The model under review builds one solid part; all positions refer to its coordinate system, in mm. A direction names the side the tool comes from. Give positions to 0.01 mm unless a question says otherwise; leave off trailing zeros. Loops run counter-clockwise (first coordinate to the right, second up) from the corner with the lowest first, then second, coordinate; pieces in that order, holes last. Notation, with made-up numbers: M 82.5,-11.5 L 114.5,-11.5 A15 cw 114.5,12.5 Z; hole C 15.5,62.25 d1. An arc over 180 degrees is marked long. Put each result on its own line as item: value. Start each with the question number.
```python
from build123d import *

# Parameters (mm, degrees)
BOSS_EXTRUDE1_DEPTH = 5


with BuildPart() as part:
    # Sketch2 → Boss-Extrude1 (new body)
    with BuildSketch(Plane(origin=(0, 0, 0), x_dir=(1, 0, 0), z_dir=(0, 1, 0))):
        with BuildLine():
            Line((-46.361864593, 80.672065662), (46.361864593, 80.672065662))
            Line((46.361864593, 80.672065662), (66.733304285, 94.936301299))
            ThreePointArc((66.733304285, 94.936301299), (74.205550425, 96.592858386), (80.660589091, 92.480545219))
            Line((80.660589091, 92.480545219), (89.264235636, 80.193264555))
            ThreePointArc((89.264235636, 80.193264555), (90.920792724, 72.721018415), (86.808479557, 66.265979749))
            Line((86.808479557, 66.265979749), (62.402393643, 49.176654414))
            ThreePointArc((62.402393643, 49.176654414), (59.268049675, 45.602620103), (58.138158007, 40.985133971))
            Line((58.138158007, 40.985133971), (58.138158007, 16.396474982))
            ThreePointArc((58.138158007, 16.396474982), (57.008266339, 11.77898885), (53.873922371, 8.204954539))
            Line((53.873922371, 8.204954539), (41.764235636, -0.274339397))
            ThreePointArc((41.764235636, -0.274339397), (38.629891668, -3.848373708), (37.5, -8.46585984))
            Line((37.5, -8.46585984), (37.5, -283.0815533))
            ThreePointArc((37.5, -283.0815533), (38.82037806, -288.047856048), (42.432832597, -291.702679358))
            Line((42.432832597, -291.702679358), (110.719624802, -331.839038015))
            ThreePointArc((110.719624802, -331.839038015), (114.964915466, -336.816247945), (115.224929316, -343.352875846))
            Line((115.224929316, -343.352875846), (110.804845639, -357.979679412))
            ThreePointArc((110.804845639, -357.979679412), (105.193270142, -364.269086107), (96.767619692, -364.034926706))
            Line((96.767619692, -364.034926706), (4.46475403, -317.978659754))
            ThreePointArc((4.46475403, -317.978659754), (0, -316.92661882), (-4.46475403, -317.978659754))
            Line((-4.46475403, -317.978659754), (-96.767619692, -364.034926706))
            ThreePointArc((-96.767619692, -364.034926706), (-105.193270142, -364.269086107), (-110.804845639, -357.979679412))
            Line((-110.804845639, -357.979679412), (-115.224929316, -343.352875846))
            ThreePointArc((-115.224929316, -343.352875846), (-114.964915466, -336.816247945), (-110.719624802, -331.839038015))
            Line((-110.719624802, -331.839038015), (-42.432832597, -291.702679358))
            ThreePointArc((-42.432832597, -291.702679358), (-38.82037806, -288.047856048), (-37.5, -283.0815533))
            Line((-37.5, -283.0815533), (-37.5, -8.46585984))
            ThreePointArc((-37.5, -8.46585984), (-38.629891668, -3.848373708), (-41.764235636, -0.274339397))
            Line((-41.764235636, -0.274339397), (-53.873922371, 8.204954539))
            ThreePointArc((-53.873922371, 8.204954539), (-57.008266339, 11.77898885), (-58.138158007, 16.396474982))
            Line((-58.138158007, 16.396474982), (-58.138158007, 40.985133971))
            ThreePointArc((-58.138158007, 40.985133971), (-59.268049675, 45.602620103), (-62.402393643, 49.176654414))
            Line((-62.402393643, 49.176654414), (-86.808479557, 66.265979749))
            ThreePointArc((-86.808479557, 66.265979749), (-90.920792724, 72.721018415), (-89.264235636, 80.193264555))
            Line((-89.264235636, 80.193264555), (-80.660589091, 92.480545219))
            ThreePointArc((-80.660589091, 92.480545219), (-74.205550425, 96.592858386), (-66.733304285, 94.936301299))
            Line((-66.733304285, 94.936301299), (-46.361864593, 80.672065662))
        make_face()
    extrude(amount=BOSS_EXTRUDE1_DEPTH)


solid = part.part
```
Item 1: Consider section B-B, the plane x = -13. Write out the cut boundary in (y, z), plus the area to 3 significant figures.
Item 2: Draft analysis for pull direction X (two halves, no side actions). For faces 6 (the flat face through (-74.43, 2.46, -57.6)), 7 (the flat face through (-56.69, 2.465, -87.904)), 8 (the flat face through (56.4, 2.5, -87.7)), 9 (the flat face through (2, 0, 131)), state which applies: +X half, -X half, draft (parallel to the pull), parting line (faces both ways), or undercut.
Item 3: Clearance check with flat-ended pins moving along their axes: pin 1 Ø1.5 at (x, y) = (59, 2.5) entering from +Z; pin 2 Ø2.5 at (y, z) = (2.5, -32) entering from +X; pin 3 Ø2.5 at (y, z) = (1.5, 78) entering from -X; pin 4 Ø10 at (x, z) = (47, 146) entering from +Y. State where each tip first meets the part, or that it passes through.
Item 4: Consider section A-A, the plane z = -25.5. Write out the cut boundary in (x, y), plus the area to 3 significant figures.
Item 5: To check wall thickness, follow L1, parallel to X at y = 0.3, z = 137; L2, parallel to X at y = 2.5, z = -29; L3, parallel to Z at x = -38.5, y = 3.3. State the ranges of each line that lie inside material, in increasing order. Write a range as [from, to].
Item 6: Tool access review of faces 1 (the flat face through (-47.734, 2.465, -3.906)), 2 (the flat face through (2, 5, 131)), 3 (the flat face through (84.902, 2.465, -86.423)), 4 (the flat face through (51.26, 2.46, 341.33)), 5 (the flat face through (47.9, 2.46, -4.02)): name each direction out of +Z, -Z, +X, -X, +Y, -Y from which nothing blocks a thin tool from reaching the whole face with its end or side.
Report:
1. outline: M 0,-80.67 L 5,-80.67 L 5,322.24 L 0,322.24 Z
1. area: 2,010 mm²
2. face 6: -X half
2. face 7: undercut
2. face 8: undercut
2. face 9: draft
3. pin 1: z = 345.56
3. pin 2: x = 58.14
3. pin 3: x = -37.5
3. pin 4: through
4. outline: M -58.14,0 L 58.14,0 L 58.14,5 L -58.14,5 Z
4. area: 581 mm²
5. L1: [-37.5, 37.5]
5. L2: [-58.14, 58.14]
5. L3: [-80.67, 4.11], [287.44, 334.96]
6. face 1: -X, +Y, -Y
6. face 2: +Z, -Z, +X, -X, +Y
6. face 3: -Z, +X, +Y, -Y
6. face 4: +Z, +Y, -Y
6. face 5: +X, +Y, -Y
